Read the model definition and answer for the solid it produces. Units are mm, in the model's axes. Round coordinates to 2 decimals unless told otherwise and drop trailing zeros. Loops run counter-clockwise (first coordinate to the right, second up) from the corner with the lowest first, then second, coordinate; pieces in that order, holes last. Notation, with made-up numbers: (83, 51) - (114, 51) arc R11 ccw to (114, 71) - close; hole circle Ø7 at (77.25, 84.5). An arc over 180 degrees is marked (long way). Use one line per item in the form item = value. Start each with the question number.
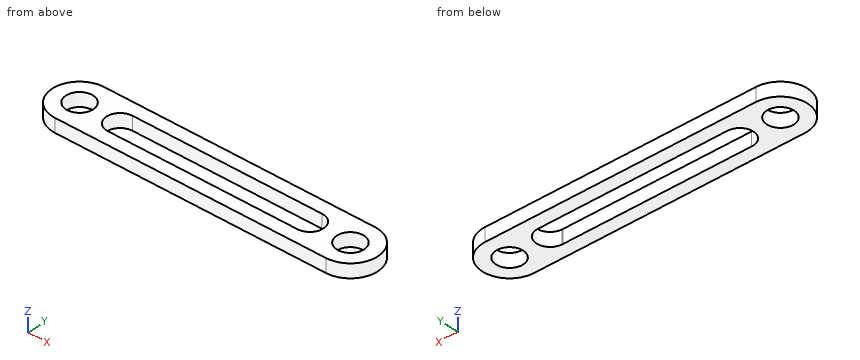
```python
from build123d import *

# Parameters (mm, degrees)
F0_R     = 5
F1_DEPTH = 5


with BuildPart() as f1:
    # F0 (on Top) → F1 (new body)
    with BuildSketch(Plane.XY):
        with BuildLine():
            Line((100, 10), (0, 10))
            ThreePointArc((0, 10), (-10, 0), (0, -10))
            Line((0, -10), (100, -10))
            ThreePointArc((100, -10), (110, 0), (100, 10))
        make_face()
        Circle(F0_R, mode=Mode.SUBTRACT)
        with BuildLine():
            ThreePointArc((15.175696, -4.996912), (10.000772, -0.087862), (15, 5))
            Line((15, 5), (85, 5))
            ThreePointArc((85, 5), (89.999228, 0.087862), (85.175696, -4.996912))
            ThreePointArc((85.175696, -4.996912), (85, -5), (84.824304, -4.996912))
            Line((84.824304, -4.996912), (15.175696, -4.996912))
        make_face(mode=Mode.SUBTRACT)
        with Locations((100, 0)):
            Circle(F0_R, mode=Mode.SUBTRACT)
    extrude(amount=F1_DEPTH)


solid = f1.part
```
1) A cutting plane is placed at D-D on x = 64. Write down the section's boundary in (y, z), plus the area to 3 significant figures.
2) A cutting plane is placed at C-C on z = 4.2. Write down the section's boundary in (x, y), plus the area to 3 significant figures.
3) A cutting plane is placed at B-B on x = 12. Write down the section's boundary in (y, z), plus the area to 3 significant figures.
4) A flat-ended cylindrical pin translates along its axis: pin 1 (11.5 mm diameter, centred on x = 100, y = 0, fed in from +Z). Find the tip coordinate at first contact, or state that the pin passes through.
5) Straight lines are drawn through the part: line 1 (Y direction, x = 33, z = 4); line 2 (X direction, y = -1.5, z = 2.1); line 3 (X direction, y = -1, z = 4.7). For each, find the intervals that lie inside material, in ascending order. Write a range as from..to.
6) A cutting plane is placed at A-A on y = 0. Write down the section's boundary in (x, z), plus the area to 4 significant figures.
Checks:
q1.outline = (-10, 0) - (-5, 0) - (-5, 5) - (-10, 5) - close; (5, 0) - (10, 0) - (10, 5) - (5, 5) - close
q1.area = 50.0 mm²
q2.outline = (0, -10) - (100, -10) arc R10 ccw to (100, 10) - (0, 10) arc R10 ccw to start; hole circle Ø10 at (0, 0); hole (15, 5) arc R5 ccw (long way) to (15.18, -5) - (84.82, -5) arc R5 ccw to (85.18, -5) arc R5 ccw to (85, 5) - close; hole circle Ø10 at (100, 0)
q2.area = 1,380 mm²
q3.outline = (-10, 0) - (-4, 0) - (-4, 5) - (-10, 5) - close; (4, 0) - (10, 0) - (10, 5) - (4, 5) - close
q3.area = 60.0 mm²
q4.pin_1 = 5
q5.line_1 = -10..-5, 5..10
q5.line_2 = -9.89..-4.77, 4.77..10.23, 89.77..95.23, 104.77..109.89
q5.line_3 = -9.95..-4.9, 4.9..10.1, 89.9..95.1, 104.9..109.95
q6.outline = (-10, 0) - (-5, 0) - (-5, 5) - (-10, 5) - close; (5, 0) - (10, 0) - (10, 5) - (5, 5) - close; (90, 0) - (95, 0) - (95, 5) - (90, 5) - close; (105, 0) - (110, 0) - (110, 5) - (105, 5) - close
q6.area = 100.0 mm²
